Source: CAD feature listing. Evaluate the final solid. Frame: model axes, mm. A direction names the side the tool comes from. Round coordinates to 2 decimals unless told otherwise and drop trailing zeros. Write each loop counter-clockwise with the first axis right and the second up, starting at its lowest first coordinate (ties: lowest second). Pieces come first, ordered by that corner, then holes. Notation, with made-up numbers: M 88.25,53 L 132.25,53 A25 ccw 132.25,69 Z; hole C 69.25,46 d9. An arc over 180 degrees is marked long. Use a Markdown table: item, result.
```python
from build123d import *
from build123d.topology import SkipClean

# Parameters (mm, degrees)
SCHIZZO1_W                   = 40.53
SCHIZZO1_H                   = 19.84
ESTRUSIONE_ESTRUSIONE1_DEPTH = 17
SCHIZZO2_W                   = 40.53
SCHIZZO2_H                   = 19.84
ESTRUSIONE_ESTRUSIONE2_DEPTH = 6.5
ESTRUSIONE_ESTRUSIONE2_TAPER = 15
SCHIZZO3_W                   = 40.58
SCHIZZO3_H                   = 20.12
ESTRUSIONE_ESTRUSIONE3_DEPTH = 7.5
SCHIZZO5_W                   = 30.52
SCHIZZO5_H                   = 20.12
ESTRUSIONE_ESTRUSIONE4_DEPTH = 4.5
SCHIZZO6_R                   = 6.035
ESTRUSIONE_ESTRUSIONE5_DEPTH = 1.5
SCHIZZO7_R                   = 2.9
ESTRUSIONE_ESTRUSIONE6_DEPTH = 4
SMUSSO1_SIZE                 = 4.5
ESTRUSIONE_ESTRUSIONE7_DEPTH = 2.5
SCHIZZO11_W                  = 6.81
SCHIZZO11_H                  = 8.89
SCHIZZO11_R                  = 2.15
ESTRUSIONE_ESTRUSIONE8_DEPTH = 1.99


with BuildPart() as part:
    # Schizzo1 → Estrusione-Estrusione1 (new body)
    with BuildSketch(Plane(origin=(0, 0, 0), x_dir=(1, 0, 0), z_dir=(0, 1, 0))):
        Rectangle(SCHIZZO1_W, SCHIZZO1_H)
    extrude(amount=ESTRUSIONE_ESTRUSIONE1_DEPTH)

    # Schizzo2 → Estrusione-Estrusione2 (add)
    with BuildSketch(Plane(origin=(0, 17, 0), x_dir=(1, 0, 0), z_dir=(0, 1, 0))):
        Rectangle(SCHIZZO2_W, SCHIZZO2_H)
    extrude(amount=ESTRUSIONE_ESTRUSIONE2_DEPTH, taper=ESTRUSIONE_ESTRUSIONE2_TAPER)

    # Schizzo3 → Estrusione-Estrusione3 (add)
    with BuildSketch(Plane(origin=(0, 0, 0), x_dir=(-1, 0, 0), z_dir=(0, -1, 0))):
        Rectangle(SCHIZZO3_W, SCHIZZO3_H)
    extrude(amount=ESTRUSIONE_ESTRUSIONE3_DEPTH)

    # Schizzo5 → Estrusione-Estrusione4 (add)
    with BuildSketch(Plane.XZ.offset(7.5)):
        with BuildLine():
            Line((10.23, -10.06), (10.23, 10.06))
            ThreePointArc((10.23, 10.06), (20.29, 0), (10.23, -10.06))
        make_face()
        with Locations((-5.03, 0)):
            Rectangle(SCHIZZO5_W, SCHIZZO5_H)
    extrude(amount=ESTRUSIONE_ESTRUSIONE4_DEPTH)

    # Schizzo6 → Estrusione-Estrusione5 (add)
    with BuildSketch(Plane.XZ.offset(12)):
        with Locations(Location((9.755, 0, 0), (0, 0, 270))):
            Circle(SCHIZZO6_R)
    extrude(amount=ESTRUSIONE_ESTRUSIONE5_DEPTH)

    # Schizzo7 → Estrusione-Estrusione6 (add)
    with BuildSketch(Plane.XZ.offset(13.5)):
        with Locations(Location((9.755, 0, 0), (0, 0, 270))):
            Circle(SCHIZZO7_R)
    extrude(amount=ESTRUSIONE_ESTRUSIONE6_DEPTH)

    # Smusso1
    smusso1_edges = [part.edges().sort_by_distance(p)[0] for p in [
        (-20.29, -12, 0),
    ]]
    chamfer(smusso1_edges, length=SMUSSO1_SIZE)

    # Schizzo8 → Estrusione-Estrusione7 (add)
    with BuildSketch(Plane(origin=(0, -3.5, 0), x_dir=(1, 0, 0), z_dir=(0, 1, 0))):
        with BuildLine():
            Line((-27.29, -10.06), (-20.29, -10.06))
            Line((-20.29, -10.06), (-20.29, 10.06))
            Line((-20.29, 10.06), (-27.29, 10.06))
            Line((-27.29, 10.06), (-27.29, 6.2))
            Line((-27.29, 6.2), (-26.283956277, 6.2))
            ThreePointArc((-26.283956277, 6.2), (-23.872706606, 7.056453986), (-22.35, 5))
            ThreePointArc((-22.35, 5), (-23.872706606, 2.943546014), (-26.283956277, 3.8))
            Line((-26.283956277, 3.8), (-27.29, 3.8))
            Line((-27.29, 3.8), (-27.29, -3.8))
            Line((-27.29, -3.8), (-26.283956277, -3.8))
            ThreePointArc((-26.283956277, -3.8), (-23.872706606, -2.943546014), (-22.35, -5))
            ThreePointArc((-22.35, -5), (-23.872706606, -7.056453986), (-26.283956277, -6.2))
            Line((-26.283956277, -6.2), (-27.29, -6.2))
            Line((-27.29, -6.2), (-27.29, -10.06))
        make_face()
        with BuildLine():
            Line((20.29, -10.06), (27.29, -10.06))
            Line((27.29, -10.06), (27.29, -6.2))
            Line((27.29, -6.2), (26.283956277, -6.2))
            ThreePointArc((26.283956277, -6.2), (22.35, -5), (26.283956277, -3.8))
            Line((26.283956277, -3.8), (27.29, -3.8))
            Line((27.29, -3.8), (27.29, 3.8))
            Line((27.29, 3.8), (26.283956277, 3.8))
            ThreePointArc((26.283956277, 3.8), (22.35, 5), (26.283956277, 6.2))
            Line((26.283956277, 6.2), (27.29, 6.2))
            Line((27.29, 6.2), (27.29, 10.06))
            Line((27.29, 10.06), (20.29, 10.06))
            Line((20.29, 10.06), (20.29, -10.06))
        make_face()
    extrude(amount=-ESTRUSIONE_ESTRUSIONE7_DEPTH)

    # Schizzo11 → Estrusione-Estrusione8 (add, symmetric)
    # profile 1 of 2: a face of its own
    with BuildSketch(Plane(origin=(0, -4.75, 0), x_dir=(-1, 0, 0), z_dir=(0, -1, 0))):
        with Locations((24.5, 5)):
            Rectangle(SCHIZZO11_W, SCHIZZO11_H)
        with Locations(Location((24.5, 5, 0), (0, 0, 90))):
            Circle(SCHIZZO11_R, mode=Mode.SUBTRACT)
    # profile 2 of 2: a face of its own
    with BuildSketch(Plane(origin=(0, -4.75, 0), x_dir=(-1, 0, 0), z_dir=(0, -1, 0))):
        with Locations((24.5, -5)):
            Rectangle(SCHIZZO11_W, SCHIZZO11_H)
        with Locations(Location((24.5, -5, 0), (0, 0, 90))):
            Circle(SCHIZZO11_R, mode=Mode.SUBTRACT)
    estrusione_estrusione8 = extrude(amount=ESTRUSIONE_ESTRUSIONE8_DEPTH, both=True)

    # Specchia1: Estrusione-Estrusione8 across plane
    with SkipClean():  # the faces are left unmerged after this step: merging them gives an invalid solid
        add(estrusione_estrusione8.mirror(Plane(origin=(0, 0, 0), x_dir=(0, 0, 1), z_dir=(1, 0, 0))))


solid = part.part
```
Q1. Section C-C on y = -1. Return loops of the section in (x, z).
Results are:
| item | result |
|---|---|
| outline | M -20.29,-10.06 L 20.29,-10.06 L 20.29,10.06 L -20.29,10.06 Z |
Q2. Section B-B on z = -5. Give the number of separate pieces and of enclosed holes in the cut face, plus the area to 3 significant figures.
Results are:
| item | result |
|---|---|
| separate pieces | 3 |
| enclosed holes | 0 |
| area | 1,450 mm^2 |
Q3. Reachability of faces 1 (the flat face through (20.29, -7, 0)), 2 (the cylindrical face through (20.288, -9.718, 0.221)), 3 (the flat face through (-22, -6.74, -5)), 4 (the flat face through (-22, -2.76, 5)), 5 (the cylindrical face through (11.71, -15.47, 2.14)) from +Z, -Z, +X, -X, +Y, -Y: full face, straight path, thin tool, end or side. Return the list, or none.
Results are:
| item | result |
|---|---|
| face 1 | +Z, -Z, -Y |
| face 2 | +X, -Y |
| face 3 | +Z, -Z, -X, -Y |
| face 4 | +Z, -Z, -X, +Y |
| face 5 | -Y |
Q4. First-contact query: pin 1 Ø3 at (x, y) = (-12.5, 4) entering from +Z; pin 2 Ø12 at (x, z) = (-15, -7.5) entering from -Y; pin 3 Ø5.5 at (x, z) = (-22.5, 0.5) entering from -Y; pin 4 Ø6 at (x, y) = (-5.5, -13.5) entering from +Z. Flat tips, straight axial feed; report the tip coordinate or a pass-through.
Results are:
| item | result |
|---|---|
| pin 1 | z = 9.92 |
| pin 2 | y = -12 |
| pin 3 | y = -8.04 |
| pin 4 | z = 10.06 |
Q5. Line query: L1, parallel to X at y = -4, z = -5 (3 decimals); L2, parallel to Z at x = -24, y = -4; L3, parallel to Y at x = -13.5, z = -4. Output: solid intervals per line, ascending.
Results are:
| item | result |
|---|---|
| L1 | -27.905 to -26.65, -22.35 to 22.35, 26.65 to 27.905 |
| L2 | -10.06 to -7.09, -2.91 to 2.91, 7.09 to 10.06 |
| L3 | -12 to 23.5 |
Q6. Section A-A on y = 15.5. Return loops of the section in (x, z) (3 decimals).
Results are:
| item | result |
|---|---|
| outline | M -20.265,-9.92 L 20.265,-9.92 L 20.265,9.92 L -20.265,9.92 Z |
